```python
from build123d import *

# Parameters (mm, degrees)
EXTRUDE_1_DEPTH     = 25
FILLET_1_R          = 10
FILLET_2_R          = 1
SKETCH_2_R          = 3.5
CUT_EXTRUDE_2_DEPTH = 25
SKETCH_4_R          = 3.5
CUT_EXTRUDE_3_DEPTH = 25


with BuildPart() as part:
    # 스케치1 → 보스-돌출1 (new body)
    with BuildSketch(Plane.XY):
        Polygon((-30, 30), (30, 30), (30, -30), (26, -26), (26, -2), (-2, 26), (-26, 26), align=None)
        Polygon((26, 26), (26, 3.656854249), (3.656854249, 26), align=None, mode=Mode.SUBTRACT)
    extrude(amount=EXTRUDE_1_DEPTH)

    # 필렛1
    fillet_1_edges = [part.edges().sort_by_distance(p)[0] for p in [
        (26, -26, 12.5),
        (-26, 26, 12.5),
    ]]
    fillet(fillet_1_edges, radius=FILLET_1_R)

    # 필렛2
    fillet_2_edges = [part.edges().sort_by_distance(p)[0] for p in [
        (26, -2, 12.5),
        (-2, 26, 12.5),
        (26, 26, 12.5),
        (3.656854249, 26, 12.5),
        (26, 3.656854249, 12.5),
    ]]
    fillet(fillet_2_edges, radius=FILLET_2_R)

    # 스케치2 → 컷-돌출2 (cut)
    with BuildSketch(Plane(origin=(0, 30, 0), x_dir=(1, 0, 0), z_dir=(0, 1, 0))):
        with Locations((-15, -12.5)):
            Circle(SKETCH_2_R)
    extrude(amount=-CUT_EXTRUDE_2_DEPTH, mode=Mode.SUBTRACT)

    # 스케치4 → 컷-돌출3 (cut)
    with BuildSketch(Plane(origin=(30, 0, 0), x_dir=(0, 0, -1), z_dir=(1, 0, 0))):
        with Locations((-12.5, -15)):
            Circle(SKETCH_4_R)
    extrude(amount=-CUT_EXTRUDE_3_DEPTH, mode=Mode.SUBTRACT)


solid = part.part
```
Design review of the part built by this model. Coordinates are the model's own, in mm. A direction names the side the tool comes from. Coordinates: 2 decimals unless noted, no trailing zeros. Order: outer loops, then holes, each group sorted by start corner. A loop starts at its lowest first (then second) coordinate and runs counter-clockwise, first axis right, second up. Notation, with made-up numbers: (-25, 62.25) - (-11, 62.25) arc R33 ccw to (-11, 97.25) - close; hole circle Ø6 at (85, 1.25). An arc over 180 degrees is marked (long way). Answer in a Markdown table with one row per item.
(1) Consider section A-A on z = 12.5. State the section outline as (x, y) points, plus the area to 3 significant figures.
Checked values:
| item | result |
|---|---|
| outline | (-30, 30) - (-28.93, 28.93) arc R10 ccw to (-21.86, 26) - (-18.5, 26) - (-18.5, 30) - close; (-11.5, 26) - (-2.41, 26) arc R1 cw to (-1.71, 25.71) - (25.71, -1.71) arc R1 cw to (26, -2.41) - (26, -11.5) - (30, -11.5) - (30, 30) - (-11.5, 30) - close; (26, -21.86) arc R10 ccw to (28.93, -28.93) - (30, -30) - (30, -18.5) - (26, -18.5) - close; hole (5.36, 24.29) - (24.29, 5.36) arc R1 ccw to (26, 6.07) - (26, 25) arc R1 ccw to (25, 26) - (6.07, 26) arc R1 ccw to start |
| area | 533 mm^2 |
(2) For faces 1 (the flat face through (30, 0, 12)), 2 (the flat face through (14.961, 14.696, 12.325)), 3 (the flat face through (-10, 26, 12)), list the 3-axis set-ups (+Z, -Z, +X, -X, +Y, -Y) from which the entire face can be reached by the end or side of a thin tool; tool diameter is ignored.
Checked values:
| item | result |
|---|---|
| face 1 | +Z, -Z, +X, +Y, -Y |
| face 2 | +Z, -Z |
| face 3 | +Z, -Z, -X, -Y |
(3) Wall thickness on line 1 along Z through (x, y) = (-15, 28.65); line 2 along Y through (x, z) = (21.5, 11); line 3 along X through (y, z) = (12, 15.25): over which ranges is each line inside the solid? List them lowest first. Write a range as from..to.
Checked values:
| item | result |
|---|---|
| line 1 | 0..9, 16..25 |
| line 2 | 2.5..8.16, 26..30 |
| line 3 | 12..17.66, 26..30 |
(4) Consider section B-B on y = -15. State the section outline as (x, z) points.
Checked values:
| item | result |
|---|---|
| outline | (26, 0) - (30, 0) - (30, 9) - (26, 9) - close; (26, 16) - (30, 16) - (30, 25) - (26, 25) - close |
(5) Consider section D-D on z = 19. State the section outline as (x, y) points, plus the area to 3 significant figures.
Checked values:
| item | result |
|---|---|
| outline | (-30, 30) - (-28.93, 28.93) arc R10 ccw to (-21.86, 26) - (-2.41, 26) arc R1 cw to (-1.71, 25.71) - (25.71, -1.71) arc R1 cw to (26, -2.41) - (26, -21.86) arc R10 ccw to (28.93, -28.93) - (30, -30) - (30, 30) - close; hole (5.36, 24.29) - (24.29, 5.36) arc R1 ccw to (26, 6.07) - (26, 25) arc R1 ccw to (25, 26) - (6.07, 26) arc R1 ccw to start |
| area | 589 mm^2 |
(6) The part is to be moulded in two halves that separate along Z. For faces 4 (the cylindrical face through (25.398, 5.154, 12.675)), 5 (the flat face through (13, 13, 25)), 6 (the cylindrical face through (-13.385, 28.028, 15.605)), say which applies: released by +Z, released by -Z, zero draft, split by the parting line, or undercut.
Checked values:
| item | result |
|---|---|
| face 4 | zero draft |
| face 5 | released by +Z |
| face 6 | undercut |
(7) Clearance check with flat-ended pins moving along their axes: pin 1 (3 mm diameter, centred on x = -6.5, z = 13, fed in from -Y); pin 2 (11 mm diameter, centred on y = -15, z = 12.5, fed in from +X); pin 3 (9.5 mm diameter, centred on x = 11.5, z = 9.5, fed in from -Y); pin 4 (15 mm diameter, centred on y = 16, z = 14.5, fed in from -X). State where each tip first meets the part, or that it passes through.
Checked values:
| item | result |
|---|---|
| pin 1 | y = 26 |
| pin 2 | x = 30 |
| pin 3 | y = 7.75 |
| pin 4 | x = 0.5 |
